```python
from build123d import *

# Parameters (mm, degrees)
SKETCH1_R           = 2.5
BOSS_EXTRUDE1_DEPTH = 300
FILLET1_R           = 1
FILLET2_R           = 0.5
FILLET3_R           = 0.5
FILLET4_R           = 0.5
FILLET5_R           = 0.5


with BuildPart() as part:
    # Sketch1 → Boss-Extrude1 (new body)
    with BuildSketch(Plane.XY):
        Polygon((13.2, 0), (13.2, 1.8), (15.45, 1.8), (15.45, 3.6), (12.95, 6.1), (7.05, 6.1), (4.55, 3.6), (4.55, 1.8), (6.8, 1.8), (6.8, 0), (0, 0), (0, 6.8), (1.8, 6.8), (1.8, 4.55), (3.6, 4.55), (6.1, 7.05), (6.1, 12.95), (3.6, 15.45), (1.8, 15.45), (1.8, 13.2), (0, 13.2), (0, 20), (6.8, 20), (6.8, 18.2), (4.55, 18.2), (4.55, 16.4), (7.05, 13.9), (12.95, 13.9), (15.45, 16.4), (15.45, 18.2), (13.2, 18.2), (13.2, 20), (20, 20), (20, 13.2), (18.2, 13.2), (18.2, 15.45), (16.4, 15.45), (13.9, 12.95), (13.9, 7.05), (16.4, 4.55), (18.2, 4.55), (18.2, 6.8), (20, 6.8), (20, 0), align=None)
        with Locations((10, 10)):
            Circle(SKETCH1_R, mode=Mode.SUBTRACT)
    boss_extrude1 = extrude(amount=BOSS_EXTRUDE1_DEPTH)

    # Fillet1
    fillet1_edges = [part.edges().sort_by_distance(p)[0] for p in [
        (0, 0, 150),
        (0, 20, 150),
        (20, 20, 150),
        (20, 0, 150),
    ]]
    fillet(fillet1_edges, radius=FILLET1_R)

    # Fillet2
    fillet2_edges = [part.edges().sort_by_distance(p)[0] for p in [
        (4.55, 18.2, 150),
        (4.55, 16.4, 150),
        (7.05, 13.9, 150),
        (12.95, 13.9, 150),
        (15.45, 16.4, 150),
        (15.45, 18.2, 150),
    ]]
    fillet(fillet2_edges, radius=FILLET2_R)

    # Fillet3
    fillet3_edges = [part.edges().sort_by_distance(p)[0] for p in [
        (18.2, 15.45, 150),
        (16.4, 15.45, 150),
        (13.9, 12.95, 150),
        (13.9, 7.05, 150),
        (16.4, 4.55, 150),
        (18.2, 4.55, 150),
    ]]
    fillet(fillet3_edges, radius=FILLET3_R)

    # Fillet4
    fillet4_edges = [part.edges().sort_by_distance(p)[0] for p in [
        (1.8, 4.55, 150),
        (3.6, 4.55, 150),
        (6.1, 7.05, 150),
        (6.1, 12.95, 150),
        (3.6, 15.45, 150),
        (1.8, 15.45, 150),
    ]]
    fillet(fillet4_edges, radius=FILLET4_R)

    # Fillet5
    fillet5_edges = [part.edges().sort_by_distance(p)[0] for p in [
        (15.45, 1.8, 150),
        (15.45, 3.6, 150),
        (12.95, 6.1, 150),
        (7.05, 6.1, 150),
        (4.55, 3.6, 150),
        (4.55, 1.8, 150),
    ]]
    fillet(fillet5_edges, radius=FILLET5_R)

    # Mirror1: Boss-Extrude1 across plane
    add(boss_extrude1.mirror(Plane(origin=(0, 0, 0), x_dir=(0, 0, 1), z_dir=(1, 0, 0))))


solid = part.part
```
Can you work these out from the model? Positions are in its coordinate system, mm. A direction names the side the tool comes from. Coordinates: 2 decimals unless noted, no trailing zeros. Loops run counter-clockwise (first coordinate to the right, second up) from the corner with the lowest first, then second, coordinate; pieces in that order, holes last. Notation, with made-up numbers: (36.5, -12) -> (67.5, -12) arc R14 ccw to (67.5, -3) -> close; hole circle Ø7 at (64, 1). An arc over 180 degrees is marked (long way). Put each result on its own line as item: value. Start each with the question number.
Q1. I want a section at C-C (z = 252.5). Count the separate pieces of the cut face and the enclosed holes in it, plus the area to 3 significant figures.
Q2. I want a section at A-A (x = 10). Write out the boundary of the cut face in (y, z).
Q3. I want a section at B-B (y = 10). Write out the boundary of the cut face in (x, z), plus the area to 3 significant figures.
Q4. Thinking about a two-plate mould opening in X: for faces 4 (the face through (20, 16, 148)), 5 (the face through (0, 15, 300)), 6 (the face through (10, 13.9, 148)), which applies, pulls with the +X half, pulls with the -X half, needs draft (parallel to the pull), parting line crosses it, or undercut?
Q5. I'm going to push flat-ended pins straight in: P1, Ø2.5, axis at y = 9.5, z = 142, coming from the -X side; P2, Ø1.6, axis at y = 11.5, z = 76.5, coming from the +X side. Where does each tip first touch, or does it pass through?
Q6. If I drill on line 1 (Y direction, x = -6, z = 101.5); line 2 (X direction, y = 17.75, z = 228.5); line 3 (X direction, y = 18.75, z = 189.5), over which ranges is the centre line in solid material (lowest first)? Write a range as [from, to].
Q7. For faces 1 (the face through (13.9, 10, 148)), 2 (the face through (-10, 6.1, 148)), 3 (the face through (-13.9, 10, 148)), which set-ups out of +Z, -Z, +X, -X, +Y, -Y let a thin tool reach every point of the face, with its end or its side?
Taken from the geometry:
1. separate pieces: 1
1. enclosed holes: 3
1. area: 343 mm2
2. outline: (6.1, 0) -> (7.5, 0) -> (7.5, 300) -> (6.1, 300) -> close; (12.5, 0) -> (13.9, 0) -> (13.9, 300) -> (12.5, 300) -> close
3. outline: (-13.9, 0) -> (-12.5, 0) -> (-12.5, 300) -> (-13.9, 300) -> close; (-7.5, 0) -> (-6.1, 0) -> (-6.1, 300) -> (-7.5, 300) -> close; (6.1, 0) -> (7.5, 0) -> (7.5, 300) -> (6.1, 300) -> close; (12.5, 0) -> (13.9, 0) -> (13.9, 300) -> (12.5, 300) -> close
3. area: 1,680 mm2
4. face 4: pulls with the +X half
4. face 5: needs draft
4. face 6: undercut
5. P1: stops at x = -13.9
5. P2: stops at x = 13.9
6. line 1: y = [0, 1.8], [5.05, 6.95], [13.05, 14.95], [18.2, 20]
6. line 2: x = [-20, -15.45], [-4.55, 4.55], [15.45, 20]
6. line 3: x = [-20, -13.2], [-6.8, 6.8], [13.2, 20]
7. face 1: +Z, -Z, +X
7. face 2: +Z, -Z, -Y
7. face 3: +Z, -Z, -X
